```python
from build123d import *

# Parameters (mm, degrees)
SKETCH1_W           = 145
SKETCH1_H           = 155
SKETCH1_R           = 1.6
SKETCH1_W_2         = 5
SKETCH1_H_2         = 15
BOSS_EXTRUDE1_DEPTH = 8
SKETCH2_R           = 2.65
CUT_EXTRUDE1_DEPTH  = 3
SKETCH3_R           = 2.65
CUT_EXTRUDE3_DEPTH  = 3


with BuildPart() as part:
    # Sketch1 → Boss-Extrude1 (new body)
    with BuildSketch(Plane(origin=(0, 0, 0), x_dir=(1, 0, 0), z_dir=(0, 1, 0))):
        Rectangle(SKETCH1_W, SKETCH1_H)
        with Locations(Location((-60, -70.5, 0), (0, 0, 270))):
            Circle(SKETCH1_R, mode=Mode.SUBTRACT)
        with Locations(Location((-36, -70.5, 0), (0, 0, 270))):
            Circle(SKETCH1_R, mode=Mode.SUBTRACT)
        with Locations(Location((-36, -20, 0), (0, 0, 270))):
            Circle(SKETCH1_R, mode=Mode.SUBTRACT)
        with Locations(Location((-60, -20, 0), (0, 0, 270))):
            Circle(SKETCH1_R, mode=Mode.SUBTRACT)
        with Locations(Location((60, -70.5, 0), (0, 0, 270))):
            Circle(SKETCH1_R, mode=Mode.SUBTRACT)
        with Locations(Location((36, -70.5, 0), (0, 0, 270))):
            Circle(SKETCH1_R, mode=Mode.SUBTRACT)
        with Locations(Location((36, -20, 0), (0, 0, 270))):
            Circle(SKETCH1_R, mode=Mode.SUBTRACT)
        with Locations(Location((60, -20, 0), (0, 0, 270))):
            Circle(SKETCH1_R, mode=Mode.SUBTRACT)
        with Locations(Location((-67.5, 47.5, 0), (0, 0, 270))):
            Circle(SKETCH1_R, mode=Mode.SUBTRACT)
        with Locations(Location((-57.5, 47.5, 0), (0, 0, 270))):
            Circle(SKETCH1_R, mode=Mode.SUBTRACT)
        with Locations(Location((-57.5, 37.5, 0), (0, 0, 270))):
            Circle(SKETCH1_R, mode=Mode.SUBTRACT)
        with Locations(Location((-67.5, 37.5, 0), (0, 0, 270))):
            Circle(SKETCH1_R, mode=Mode.SUBTRACT)
        with Locations(Location((67.5, 47.5, 0), (0, 0, 270))):
            Circle(SKETCH1_R, mode=Mode.SUBTRACT)
        with Locations(Location((57.5, 47.5, 0), (0, 0, 270))):
            Circle(SKETCH1_R, mode=Mode.SUBTRACT)
        with Locations(Location((57.5, 37.5, 0), (0, 0, 270))):
            Circle(SKETCH1_R, mode=Mode.SUBTRACT)
        with Locations(Location((67.5, 37.5, 0), (0, 0, 270))):
            Circle(SKETCH1_R, mode=Mode.SUBTRACT)
        with Locations(Location((0, -74, 0), (0, 0, 270))):
            Circle(SKETCH1_R, mode=Mode.SUBTRACT)
        with Locations(Location((36, -49, 0), (0, 0, 270))):
            Circle(SKETCH1_R, mode=Mode.SUBTRACT)
        with Locations(Location((-36, -49, 0), (0, 0, 270))):
            Circle(SKETCH1_R, mode=Mode.SUBTRACT)
        with Locations(Location((-64.9, -42, 0), (0, 0, 270))):
            Circle(SKETCH1_R, mode=Mode.SUBTRACT)
        with Locations(Location((-64.9, 23, 0), (0, 0, 270))):
            Circle(SKETCH1_R, mode=Mode.SUBTRACT)
        with Locations(Location((0, 50, 0), (0, 0, 270))):
            Circle(SKETCH1_R, mode=Mode.SUBTRACT)
        with Locations(Location((64.9, -42, 0), (0, 0, 270))):
            Circle(SKETCH1_R, mode=Mode.SUBTRACT)
        with Locations(Location((64.9, 23, 0), (0, 0, 270))):
            Circle(SKETCH1_R, mode=Mode.SUBTRACT)
        with Locations(Location((-10, 72.5, 0), (0, 0, 270))):
            Circle(SKETCH1_R, mode=Mode.SUBTRACT)
        with Locations(Location((0, 72.5, 0), (0, 0, 270))):
            Circle(SKETCH1_R, mode=Mode.SUBTRACT)
        with Locations(Location((10, 62.5, 0), (0, 0, 270))):
            Circle(SKETCH1_R, mode=Mode.SUBTRACT)
        with Locations(Location((0, 62.5, 0), (0, 0, 270))):
            Circle(SKETCH1_R, mode=Mode.SUBTRACT)
        with Locations(Location((-10, 62.5, 0), (0, 0, 270))):
            Circle(SKETCH1_R, mode=Mode.SUBTRACT)
        with Locations(Location((10, 72.5, 0), (0, 0, 270))):
            Circle(SKETCH1_R, mode=Mode.SUBTRACT)
        with Locations((-68.4, 4)):
            Rectangle(SKETCH1_W_2, SKETCH1_H_2, mode=Mode.SUBTRACT)
        with Locations((68.4, 4)):
            Rectangle(SKETCH1_W_2, SKETCH1_H_2, mode=Mode.SUBTRACT)
    extrude(amount=BOSS_EXTRUDE1_DEPTH)

    # Sketch2 → Cut-Extrude1 (cut)
    with BuildSketch(Plane(origin=(0, 8, 0), x_dir=(1, 0, 0), z_dir=(0, 1, 0))):
        with Locations(Location((-57.5, 47.5, 0), (0, 0, 270))):
            Circle(SKETCH2_R)
        with Locations(Location((-67.5, 47.5, 0), (0, 0, 270))):
            Circle(SKETCH2_R)
        with Locations(Location((-57.5, 37.5, 0), (0, 0, 270))):
            Circle(SKETCH2_R)
        with Locations(Location((-67.5, 37.5, 0), (0, 0, 270))):
            Circle(SKETCH2_R)
        with Locations(Location((67.5, 47.5, 0), (0, 0, 90))):
            Circle(SKETCH2_R)
        with Locations(Location((57.5, 47.5, 0), (0, 0, 90))):
            Circle(SKETCH2_R)
        with Locations(Location((57.5, 37.5, 0), (0, 0, 90))):
            Circle(SKETCH2_R)
        with Locations(Location((67.5, 37.5, 0), (0, 0, 90))):
            Circle(SKETCH2_R)
        with Locations(Location((-36, -70.5, 0), (0, 0, 270))):
            Circle(SKETCH2_R)
        with Locations(Location((-60, -70.5, 0), (0, 0, 270))):
            Circle(SKETCH2_R)
        with Locations(Location((-36, -20, 0), (0, 0, 270))):
            Circle(SKETCH2_R)
        with Locations(Location((-60, -20, 0), (0, 0, 270))):
            Circle(SKETCH2_R)
        with Locations(Location((36, -70.5, 0), (0, 0, 90))):
            Circle(SKETCH2_R)
        with Locations(Location((60, -70.5, 0), (0, 0, 90))):
            Circle(SKETCH2_R)
        with Locations(Location((36, -20, 0), (0, 0, 90))):
            Circle(SKETCH2_R)
        with Locations(Location((60, -20, 0), (0, 0, 90))):
            Circle(SKETCH2_R)
    extrude(amount=-CUT_EXTRUDE1_DEPTH, mode=Mode.SUBTRACT)

    # Sketch3 → Cut-Extrude3 (cut)
    with BuildSketch(Plane(origin=(0, 0, 0), x_dir=(1, 0, 0), z_dir=(0, 1, 0))):
        with Locations(Location((0, 50, 0), (0, 0, 270))):
            Circle(SKETCH3_R)
        with Locations(Location((-64.9, 23, 0), (0, 0, 270))):
            Circle(SKETCH3_R)
        with Locations(Location((-64.9, -42, 0), (0, 0, 270))):
            Circle(SKETCH3_R)
        with Locations(Location((-36, -49, 0), (0, 0, 270))):
            Circle(SKETCH3_R)
        with Locations(Location((0, -74, 0), (0, 0, 270))):
            Circle(SKETCH3_R)
        with Locations(Location((36, -49, 0), (0, 0, 90))):
            Circle(SKETCH3_R)
        with Locations(Location((64.9, -42, 0), (0, 0, 90))):
            Circle(SKETCH3_R)
        with Locations(Location((64.9, 23, 0), (0, 0, 90))):
            Circle(SKETCH3_R)
    extrude(amount=CUT_EXTRUDE3_DEPTH, mode=Mode.SUBTRACT)


solid = part.part
```
Read the model definition and answer for the solid it produces. Units are mm, in the model's axes. A direction names the side the tool comes from. Give positions to 0.01 mm unless a question says otherwise; leave off trailing zeros. Answer as a JSON object with one key per item and string values.
1) Straight lines are drawn through the part: probe 1 along X at (y, z) = (6.3, -37.5); probe 2 along X at (y, z) = (3.75, -72.5); probe 3 along Z at (x, y) = (60, 3.05). For each, find the intervals that lie inside material, in ascending order. Write a range as from..to.
Findings below:
{"probe 1": "x = -72.5..-70.15, -64.85..-60.15, -54.85..54.85, 60.15..64.85, 70.15..72.5", "probe 2": "x = -72.5..-11.6, -8.4..-1.6, 1.6..8.4, 11.6..72.5", "probe 3": "z = -77.5..18.4, 21.6..68.9, 72.1..77.5"}
2) A tool of negligible diameter and unlimited length cuts with its end or side. For faces 1 (the cylindrical face through (66.512, 1.479, 44.103)), 2 (the cylindrical face through (-10.61, 3.94, -61.02)), 3 (the flat face through (-60, 5, 22)), from which of +Z, -Z, +X, -X, +Y, -Y can it reach the whole face along a straight path? Write none if from no direction.
Findings below:
{"face 1": "-Y", "face 2": "+Y, -Y", "face 3": "+Y"}
3) Flat-ended cylindrical pins translate along their axes: pin 1 Ø1.6 at (x, z) = (-37, 18.5) entering from +Y; pin 2 Ø5 at (x, z) = (-64.9, -23) entering from -Y. Find the tip coordinate at first contact, or state that the pin passes through.
Findings below:
{"pin 1": "stops at y = 5", "pin 2": "stops at y = 3"}
4) For a pull along X with two mould halves and no side action, classify faces 4 (the flat face through (-1, 4, 77.5)), 5 (the flat face through (38, 5, 20)) as pulls with the +X half, pulls with the -X half, needs draft (parallel to the pull), parting line crosses it, or undercut.
Findings below:
{"face 4": "needs draft", "face 5": "undercut"}
5) Section A-A on y = 1.5 is taken. Count the separate pieces of the cut face and the enclosed holes in it, then the cut area to 3 significant figures.
Findings below:
{"separate pieces": "1", "enclosed holes": "32", "area": "22,000 mm^2"}
